from build123d import *
from build123d import SkipClean  # not in build123d's __all__

# Parameters (mm, degrees)
F0_W     = 2.875
F0_H     = 3
F1_DEPTH = 40
F2_DEPTH = 15
F3_DEPTH = 10
F4_DEPTH = 15
F5_DEPTH = 5


with BuildPart() as f1:
    # F0 (on Front) → F1 (new body)
    with BuildSketch(Plane.XZ):
        Polygon((-9.225, 4.615817529), (-9.225, 8.415817529), (-9.225, 11.415817529), (-9.225, 14.615817529), (9.225, 14.615817529), (9.225, 11.415817529), (9.225, 8.415817529), (9.225, 4.615817529), (14.225, 4.615817529), (14.225, 19.615817529), (5.6568542495, 19.615817529), (1.5, 19.615817529), (0, 19.615817529), (-1.5, 19.615817529), (-5.6568542495, 19.615817529), (-14.225, 19.615817529), (-14.225, 4.615817529), align=None)
        with Locations((-7.7875, 9.915817529)):
            Rectangle(F0_W, F0_H)
        with Locations((7.7875, 9.915817529)):
            Rectangle(F0_W, F0_H)
    extrude(amount=F1_DEPTH)

    # F0 (on Front) → F2 (join)
    with BuildSketch(Plane.XZ):
        with BuildLine():
            Line((-8.1629870472, 30.4060210151), (-14.225, 19.615817529))
            Line((-14.225, 19.615817529), (-5.6568542495, 19.615817529))
            ThreePointArc((-5.6568542495, 19.615817529), (-8.766648515, 24.5796756343), (-8.1629870472, 30.4060210151))
        make_face()
        with BuildLine():
            ThreePointArc((-8.1629870472, 30.4060210151), (-8.766648515, 24.5796756343), (-5.6568542495, 19.615817529))
            Line((-5.6568542495, 19.615817529), (-1.5, 19.615817529))
            Line((-1.5, 19.615817529), (-1.5, 19.7784203634))
            ThreePointArc((-1.5, 19.7784203634), (-4.3874821937, 32.0701735863), (7, 26.615817529))
            ThreePointArc((7, 26.615817529), (5.4543560573, 22.2283353353), (1.5, 19.7784203634))
            Line((1.5, 19.7784203634), (1.5, 19.615817529))
            Line((1.5, 19.615817529), (5.6568542495, 19.615817529))
            ThreePointArc((5.6568542495, 19.615817529), (8.7219157357, 24.3958657503), (8.3150665238, 30.0596045005))
            ThreePointArc((8.3150665238, 30.0596045005), (0.8822712117, 35.5724685498), (-7.4833147735, 31.615817529))
            Line((-7.4833147735, 31.615817529), (-8.1629870472, 30.4060210151))
        make_face()
        with BuildLine():
            Line((5.6568542495, 19.615817529), (14.225, 19.615817529))
            Line((14.225, 19.615817529), (8.3150665238, 30.0596045005))
            ThreePointArc((8.3150665238, 30.0596045005), (8.7219157357, 24.3958657503), (5.6568542495, 19.615817529))
        make_face()
    extrude(amount=F2_DEPTH)

    # F0 (on Front) → F3 (join)
    with BuildSketch(Plane.XZ):
        with BuildLine():
            ThreePointArc((-1.5, 19.7784203634), (-0.7543937436, 19.6565869623), (0, 19.615817529))
            ThreePointArc((0, 19.615817529), (0.7543937436, 19.6565869623), (1.5, 19.7784203634))
            Line((1.5, 19.7784203634), (1.5, 24.615817529))
            Line((1.5, 24.615817529), (0, 26.615817529))
            Line((0, 26.615817529), (-1.5, 24.615817529))
            Line((-1.5, 24.615817529), (-1.5, 19.7784203634))
        make_face()
        with BuildLine():
            Line((-1.5, 19.7784203634), (-1.5, 19.615817529))
            Line((-1.5, 19.615817529), (0, 19.615817529))
            ThreePointArc((0, 19.615817529), (-0.7543937436, 19.6565869623), (-1.5, 19.7784203634))
        make_face()
        with BuildLine():
            Line((0, 19.615817529), (1.5, 19.615817529))
            Line((1.5, 19.615817529), (1.5, 19.7784203634))
            ThreePointArc((1.5, 19.7784203634), (0.7543937436, 19.6565869623), (0, 19.615817529))
        make_face()
    extrude(amount=F3_DEPTH)

    # F0 (on Front) → F4 (join)
    with BuildSketch(Plane.XZ):
        with BuildLine():
            Line((0, 19.615817529), (1.5, 19.615817529))
            Line((1.5, 19.615817529), (1.5, 19.7784203634))
            ThreePointArc((1.5, 19.7784203634), (0.7543937436, 19.6565869623), (0, 19.615817529))
        make_face()
        with BuildLine():
            Line((-1.5, 19.7784203634), (-1.5, 19.615817529))
            Line((-1.5, 19.615817529), (0, 19.615817529))
            ThreePointArc((0, 19.615817529), (-0.7543937436, 19.6565869623), (-1.5, 19.7784203634))
        make_face()
    extrude(amount=F4_DEPTH)

    # F0 (on Front) → F5 (cut)
    with BuildSketch(Plane.XZ):
        with BuildLine():
            ThreePointArc((-1.5, 19.7784203634), (-0.7543937436, 19.6565869623), (0, 19.615817529))
            ThreePointArc((0, 19.615817529), (0.7543937436, 19.6565869623), (1.5, 19.7784203634))
            Line((1.5, 19.7784203634), (1.5, 24.615817529))
            Line((1.5, 24.615817529), (0, 26.615817529))
            Line((0, 26.615817529), (-1.5, 24.615817529))
            Line((-1.5, 24.615817529), (-1.5, 19.7784203634))
        make_face()
    with SkipClean():  # cleaning this boolean's faces spoils the solid; the shape is the same uncleaned
        extrude(amount=F5_DEPTH, mode=Mode.SUBTRACT)


solid = f1.part
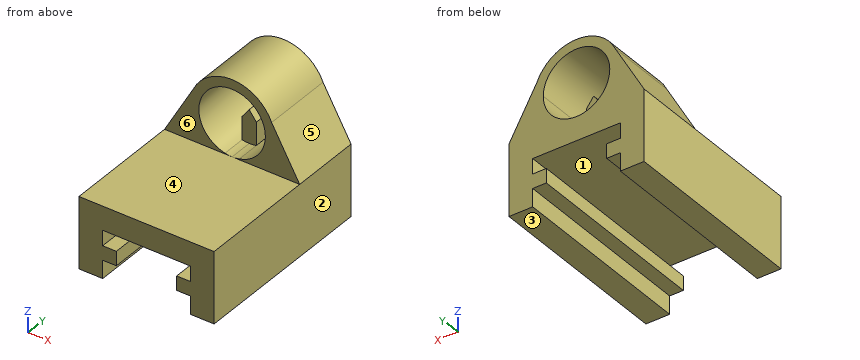
Geometry check sheet. Reference: the model listing, model coordinates, mm. Face numbers are marked on the shaded views. A direction names the side the tool comes from. Round coordinates to 2 decimals unless told otherwise and drop trailing zeros. Write each loop counter-clockwise with the first axis right and the second up, starting at its lowest first coordinate (ties: lowest second). Pieces come first, ordered by that corner, then holes. Notation, with made-up numbers: (82, 2) -> (100, 2) arc R6 cw to (100, 12) -> close; hole circle Ø2 at (-31, 89.5). An arc over 180 degrees is marked (long way). One line per item, written item: value. Start each with the question number.
(1) Go/stop test with flat-tipped pins: pin 1 Ø0.9 at (x, y) = (-7, -14) entering from +Z; pin 2 Ø8 at (x, y) = (1.5, -34.5) entering from -Z; pin 3 Ø1.5 at (x, z) = (-0.5, 23) entering from +Y; pin 4 Ø12 at (y, z) = (-22.5, 26) entering from +X. Record where each tip stops, or that it passes through.
(2) Cross-section at A-A, the plane x = 3. Record the cut outline in (y, z), and give its area (3 significant figures).
(3) Cross-section at B-B, the plane y = -23.5. Record the cut outline in (x, z) (3 decimals).
(4) Scan lines: line 1 (X direction, y = -35, z = 10) (3 decimals); line 2 (Z direction, x = 0, y = -4.5); line 3 (Z direction, x = 5.5, y = -36). Record each from-to range of solid material in increasing order. Write a range as [from, to].
(5) Cross-section at D-D, the plane z = 25.5. Record the cut outline in (x, y).
(6) Draft check along Z on the marked faces 1, 2, 3 and 4. Enter one of: +Z half, -Z half, draft (parallel to the pull), parting line (faces both ways), or undercut.
(7) Cross-section at C-C, the plane z = 31. Record the cut outline in (x, y).
(8) Access from +Z, -Z, +X, -X, +Y, -Y to the whole of each face (thin tool, end or side, straight path). Record for the marked faces 5 and 6.
Answer:
1. pin 1: z = 32.79
1. pin 2: z = 14.62
1. pin 3: y = -5
1. pin 4: through
2. outline: (-40, 14.62) -> (0, 14.62) -> (0, 20.29) -> (-15, 20.29) -> (-15, 19.62) -> (-40, 19.62) -> close; (-15, 32.94) -> (0, 32.94) -> (0, 35.1) -> (-15, 35.1) -> close
2. area: 243 mm²
3. outline: (-14.225, 4.616) -> (-9.225, 4.616) -> (-9.225, 8.416) -> (-6.35, 8.416) -> (-6.35, 11.416) -> (-9.225, 11.416) -> (-9.225, 14.616) -> (9.225, 14.616) -> (9.225, 11.416) -> (6.35, 11.416) -> (6.35, 8.416) -> (9.225, 8.416) -> (9.225, 4.616) -> (14.225, 4.616) -> (14.225, 19.616) -> (-14.225, 19.616) -> close
4. line 1: [-14.225, -6.35], [6.35, 14.225]
4. line 2: [14.62, 19.62], [33.62, 35.62]
4. line 3: [14.62, 19.62]
5. outline: (-10.92, -15) -> (-6.91, -15) -> (-6.91, 0) -> (-10.92, 0) -> close; (-0.84, -10) -> (0.84, -10) -> (0.84, -5) -> (-0.84, -5) -> close; (6.91, -15) -> (10.9, -15) -> (10.9, 0) -> (6.91, 0) -> close
6. face 1: undercut
6. face 2: draft
6. face 3: -Z half
6. face 4: +Z half
7. outline: (-7.83, -15) -> (-5.46, -15) -> (-5.46, 0) -> (-7.83, 0) -> close; (5.46, -15) -> (7.86, -15) -> (7.86, 0) -> (5.46, 0) -> close
8. face 5: +Z, +X, +Y, -Y
8. face 6: +Z, +X, -X, -Y
